Build history of the part. All positions in model axes, mm. Face numbers are marked on the shaded views. A direction names the side the tool comes from. Give positions to 0.01 mm unless a question says otherwise; leave off trailing zeros. Loops run counter-clockwise (first coordinate to the right, second up) from the corner with the lowest first, then second, coordinate; pieces in that order, holes last. Notation, with made-up numbers: (79.5, 6.5) -> (111.5, 6.5) arc R11 ccw to (111.5, 12.5) -> close; hole circle Ø8 at (7.5, -13.5). An arc over 180 degrees is marked (long way). Answer as a JSON object with one key per item and string values. Group by question number.
Q1. Wall check: probe 1 along X at (y, z) = (8.5, -2.5); probe 2 along X at (y, z) = (5.75, -5.5); probe 3 along Z at (x, y) = (33.85, 5.9). Give the ranges that are in metal, low to high. Write a range as from..to.
Q2. Drop flat-ended pins along their axis: pin 1 (0.6 mm diameter, centred on x = 36.5, y = 6.5, fed in from +Z) (3 decimals); pin 2 (1.6 mm diameter, centred on y = 6.5, z = -1.5, fed in from +X). Give the stop position or say it passes through.
Q3. Band-saw the part on A-A, the plane z = -0.5. Write the cut outline in (x, y).
Q4. Tool access for the marked faces 1, 2 and 3: list every direction of +Z, -Z, +X, -X, +Y, -Y with a clear straight run to the whole face (end or side of a thin tool).
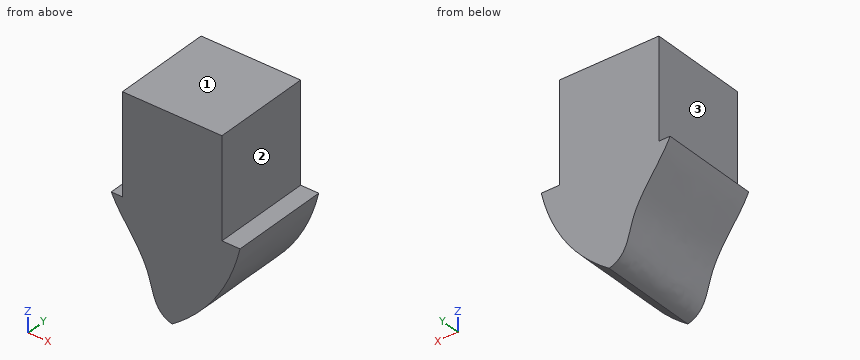
from build123d import *

# Parameters (mm, degrees)
SKETCH1_W           = 3.175
SKETCH1_H           = 3.175
BOSS_EXTRUDE1_DEPTH = 6.35
SKETCH2_W           = 6.35
SKETCH2_H           = 3.175
BOSS_EXTRUDE2_DEPTH = 3.175
CUT_EXTRUDE1_DEPTH  = 39.17066496


with BuildPart() as part:
    # Sketch1 → Boss-Extrude1 (new body)
    with BuildSketch(Plane.XY):
        with Locations((34.329620229, 7.041119721)):
            Rectangle(SKETCH1_W, SKETCH1_H)
    extrude(amount=-BOSS_EXTRUDE1_DEPTH)

    # Sketch2 → Boss-Extrude2 (add)
    with BuildSketch(Plane.XZ.offset(-5.453619721)):
        with Locations((34.329620229, -4.7625)):
            Rectangle(SKETCH2_W, SKETCH2_H)
    extrude(amount=-BOSS_EXTRUDE2_DEPTH)

    # Sketch3 → Cut-Extrude1 (cut, through all)
    with BuildSketch(Plane.XZ.offset(-5.453619721)):
        with BuildLine():
            Line((32.385431634, -3.175), (31.154620229, -3.175))
            Line((31.154620229, -3.175), (31.154620229, -6.35))
            Line((31.154620229, -6.35), (34.329620229, -6.35))
            add(Edge.make_bspline(
                [(32.385431634, -3.175), (32.718801205, -3.878392461), (33.690338088, -4.759412755), (33.756564545, -6.211143962), (34.329620229, -6.35)],
                knots=[0, 0, 0, 0, 0.611532208, 1, 1, 1, 1], degree=3))
        make_face()
        with BuildLine():
            add(Edge.make_bspline(
                [(36.495266727, -3.175), (36.021022313, -5.174773028), (34.329620229, -6.35)],
                knots=[0, 0, 0, 1, 1, 1], degree=2))
            Line((34.329620229, -6.35), (37.504620229, -6.35))
            Line((37.504620229, -6.35), (37.504620229, -3.175))
            Line((37.504620229, -3.175), (36.495266727, -3.175))
        make_face()
        Polygon((31.154620229, -3.175), (30.277564026, -3.175), (30.277564026, -6.620269694), (37.803879314, -6.620269694), (37.803879314, -3.175), (37.504620229, -3.175), (37.504620229, -6.35), (34.329620229, -6.35), (31.154620229, -6.35), align=None)
    extrude(amount=-CUT_EXTRUDE1_DEPTH, mode=Mode.SUBTRACT)


solid = part.part
Worked answers:
{
 "1": {"probe 1": "32.74..35.92", "probe 2": "33.67..35.3", "probe 3": "-5.99..0"},
 "2": {"pin 1": "z = -3.175", "pin 2": "x = 35.92"},
 "3": {"outline": "(32.74, 5.45) -> (35.92, 5.45) -> (35.92, 8.63) -> (32.74, 8.63) -> close"},
 "4": {"face 1": "+Z, +X, -X, +Y, -Y", "face 2": "+Z, +X, +Y, -Y", "face 3": "+Z, -X, +Y, -Y"}
}
